Autodesk Inventor part; units mm, degrees
ref_plane "MSC_PT1" through (0, 0, 2.7) normal (0, 0, 1) x (1, 0, 0)
ref_plane "MSC_PT2" through (0, 0, 0) normal (0, 0, -1) x (-1, 0, 0)
ref_plane "MSC_PF1" through (0, 0, 0) normal (1, 0, 0) x (0, 1, 0)
sketch "Sketch1" plane through (0, 0, 0) normal (0, 0, 1) x (1, 0, 0)
  circle A0 centre (0, 0) radius 4 construction
  line L0 (-4, 2.3094) -> (-4, -2.3094)
  line L1 (-4, -2.3094) -> (0, -4.6188)
  line L2 (0, -4.6188) -> (4, -2.3094)
  line L3 (4, -2.3094) -> (4, 2.3094)
  line L4 (4, 2.3094) -> (0, 4.6188)
  line L5 (0, 4.6188) -> (-4, 2.3094)
  line L6 (0, 6.4663) -> (0, -6.4663)
  line L7 (-5.6, 0) -> (5.6, 0)
  point P0 (0, 0)
  dimension "ParS" = 8
extrude "Extrusion1" add sketch "Sketch1" along normal blind 2.7
sketch "Sketch2" plane through (0, 0, 2.7) normal (0, 0, 1) x (1, 0, 0)
  point P0 (0, 0)
  point P1 (0, 0)
hole "Hole1" at (0, 0, 2.7) direction (0, 0, -1) diameter 4.134 end through all
ref_plane "MSC_PT1" through (0, 0, 2.7) normal (0, 0, 1) x (1, 0, 0)
ref_plane "MSC_PT2" through (0, 0, 0) normal (0, 0, -1) x (-1, 0, 0)
ref_plane "MSC_PF1" through (0, 0, 0) normal (1, 0, 0) x (0, 1, 0)
chamfer "Chamfer1" distance 0.48 angle 45 2 edges at (0, 2.067, 2.7) (0, 2.067, 0)
equation "\"d17\" = 0.6 * PTC"
equation "\"d18\" = 0.6 * PTC"
equation "\"d4\" = M"
equation "\"PTC\" = 0.8"
equation "\"NND\" = 5"
equation "\"THREADDIA\" = NND"
properties part number "CSN EN 24 036 - M5" material "Steel, Mild"
The model under review builds one solid part; all positions refer to its coordinate system, in mm. Coordinates: 2 decimals unless noted, no trailing zeros. Order: outer loops, then holes, each group sorted by start corner. A loop starts at its lowest first (then second) coordinate and runs counter-clockwise, first axis right, second up. Notation, with made-up numbers: (4, 63) -> (8, 63) arc R24 cw to (8, 97) -> close; hole circle Ø2 at (67, 60). An arc over 180 degrees is marked (long way). Answer in a Markdown table with one row per item. Add a question column.
Item 1: Mouldability with a two-part tool opening along X and no side actions: class faces 1 (the flat face through (-1.97, 3.48, 1.33)), 2 (the flat face through (2.028, 3.448, 1.331)), 3 (the flat face through (2, -2, 0)), 4 (the cylindrical face through (1.26, 1.64, 1.34)) as +X half, -X half, draft (parallel to the pull), parting line (faces both ways), or undercut.
Item 2: We need section A-A on y = 0. Write out the cut boundary in (x, z).
Item 3: To check wall thickness, follow probe 1 along X at (y, z) = (0, 1.45); probe 2 along X at (y, z) = (2, 0.25); probe 3 along Y at (x, z) = (0.25, 0.35). State the ranges of each line that lie inside material, in increasing order.
Item 4: Clearance check with a flat-ended pin moving along its axis: pin 1 (1 mm diameter, centred on x = 1.5, y = -3, fed in from -Z). State where the tip first meets the part, or that it passes through.
Item 5: We need section C-C on y = -3. Write out the cut boundary in (x, z), plus the area to 3 significant figures.
Item 6: We need section B-B on z = 1.3. Write out the cut boundary in (x, y).
Final values:
| question | item | result |
|---|---|---|
| 1 | face 1 | -X half |
| 1 | face 2 | +X half |
| 1 | face 3 | draft |
| 1 | face 4 | undercut |
| 2 | outline | (-4, 0) -> (-2.55, 0) -> (-2.07, 0.48) -> (-2.07, 2.22) -> (-2.55, 2.7) -> (-4, 2.7) -> close; (2.07, 0.48) -> (2.55, 0) -> (4, 0) -> (4, 2.7) -> (2.55, 2.7) -> (2.07, 2.22) -> close |
| 3 | probe 1 | x = -4 to -2.07, 2.07 to 4 |
| 3 | probe 2 | x = -4 to -1.13, 1.13 to 4 |
| 3 | probe 3 | y = -4.47 to -2.18, 2.18 to 4.47 |
| 4 | pin 1 | stops at z = 0 |
| 5 | outline | (-2.8, 0) -> (2.8, 0) -> (2.8, 2.7) -> (-2.8, 2.7) -> close |
| 5 | area | 15.1 mm2 |
| 6 | outline | (-4, -2.31) -> (0, -4.62) -> (4, -2.31) -> (4, 2.31) -> (0, 4.62) -> (-4, 2.31) -> close; hole circle Ø4.13 at (0, 0) |
